Autodesk Inventor part; units mm, degrees
ref_plane "Work Plane1" through (-24.15, -24.15, 49.8) normal (0, 0, 1) x (1, 0, 0)
ref_plane "YZ Plane" through (0, 0, 0) normal (1, 0, 0) x (0, 1, 0)
ref_plane "XZ Plane" through (0, 0, 0) normal (0, 1, 0) x (-1, 0, 0)
sketch "Sketch1" plane through (0, 0, 0) normal (0, 0, 1) x (1, 0, 0)
  circle A0 centre (-21.9, -21.9) radius 1.875
  circle A1 centre (21.9, 21.9) radius 1.875
  circle A2 centre (21.9, -21.9) radius 1.875
  circle A3 centre (-21.9, 21.9) radius 1.875
  circle A4 centre (14.4, 20.8) radius 2.0675
  circle A5 centre (-14.4, -20.8) radius 2.0675
  circle A6 centre (14.4, -20.8) radius 2.0675
  circle A7 centre (20.8, -14.4) radius 2.0675
  line L0 (-17.05, 17.05) -> (-17.05, -17.05)
  line L1 (17.05, 17.05) -> (-17.05, 17.05)
  line L2 (17.05, -17.05) -> (17.05, 17.05)
  line L3 (-17.05, -17.05) -> (17.05, -17.05)
  circle A8 centre (20.8, 14.4) radius 2.0675
  circle A9 centre (-14.4, 20.8) radius 2.0675
  circle A10 centre (-20.8, -14.4) radius 2.0675
  circle A11 centre (-20.8, 14.4) radius 2.0675
  line L4 (-22.9, 24.15) -> (22.9, 24.15)
  arc A12 (-22.9, 24.15) -> (-24.15, 22.9) centre (-22.9, 22.9) ccw
  line L5 (-24.15, -22.9) -> (-24.15, 22.9)
  arc A13 (-24.15, -22.9) -> (-22.9, -24.15) centre (-22.9, -22.9) ccw
  line L6 (22.9, -24.15) -> (-22.9, -24.15)
  arc A14 (22.9, -24.15) -> (24.15, -22.9) centre (22.9, -22.9) ccw
  line L7 (24.15, 22.9) -> (24.15, -22.9)
  arc A15 (24.15, 22.9) -> (22.9, 24.15) centre (22.9, 22.9) ccw
  point P0 (0, 0)
ref_plane "Work Plane1" through (-24.15, -24.15, 49.8) normal (0, 0, 1) x (1, 0, 0)
extrude "Extrusion1" add sketch "Sketch1" along normal blind 1.5 from surface at 49.8 contours A0 | A1 | A2 | A3 | L1 L2 L3 L0 | L4 A15 L7 A14 L6 A13 L5 A12
sketch "Sketch2" plane through (-22.9, -24.15, 51.3) normal (0, 0, 1) x (1, 0, 0)
  arc A0 (-1.25, 1.25) -> (0, 0) centre (0, 1.25) ccw
  line L0 (45.8, 0) -> (0, 0)
  arc A1 (45.8, 0) -> (47.05, 1.25) centre (45.8, 1.25) ccw
  line L1 (47.05, 47.05) -> (47.05, 1.25)
  arc A2 (47.05, 47.05) -> (45.8, 48.3) centre (45.8, 47.05) ccw
  line L2 (0, 48.3) -> (45.8, 48.3)
  arc A3 (0, 48.3) -> (-1.25, 47.05) centre (0, 47.05) ccw
  line L3 (-1.25, 1.25) -> (-1.25, 47.05)
  circle A4 centre (2.1, 38.55) radius 2.0675
  circle A5 centre (2.1, 9.75) radius 2.0675
  circle A6 centre (8.5, 44.95) radius 2.0675
  circle A7 centre (43.7, 38.55) radius 2.0675
  circle A8 centre (43.7, 9.75) radius 2.0675
  circle A9 centre (37.3, 3.35) radius 2.0675
  circle A10 centre (8.5, 3.35) radius 2.0675
  circle A11 centre (37.3, 44.95) radius 2.0675
  arc A12 (47.9, 47.05) -> (45.8, 49.15) centre (45.8, 47.05) ccw
  line L4 (47.9, 47.05) -> (47.9, 1.25)
  arc A13 (45.8, -0.85) -> (47.9, 1.25) centre (45.8, 1.25) ccw
  line L5 (45.8, -0.85) -> (0, -0.85)
  arc A14 (-2.1, 1.25) -> (0, -0.85) centre (0, 1.25) ccw
  line L6 (-2.1, 1.25) -> (-2.1, 47.05)
  arc A15 (0, 49.15) -> (-2.1, 47.05) centre (0, 47.05) ccw
  line L7 (0, 49.15) -> (45.8, 49.15)
  line L8 (47.05, 1.25) -> (45.8, 1.25)
  line L9 (45.8, 1.25) -> (45.8, -0.85)
  line L10 (45.8, -0.85) -> (47.05, -0.85)
  line L11 (47.05, -0.85) -> (47.05, 1.25)
  line L12 (-1.25, 1.25) -> (0, 1.25)
  line L13 (0, 1.25) -> (0, -0.85)
  line L14 (0, -0.85) -> (-1.25, -0.85)
  line L15 (-1.25, -0.85) -> (-1.25, 1.25)
  line L16 (-1.25, 47.05) -> (0, 47.05)
  line L17 (0, 47.05) -> (0, 49.15)
  line L18 (0, 49.15) -> (-1.25, 49.15)
  line L19 (-1.25, 49.15) -> (-1.25, 47.05)
  line L20 (47.05, 47.05) -> (45.8, 47.05)
  line L21 (45.8, 47.05) -> (45.8, 49.15)
  line L22 (45.8, 49.15) -> (47.05, 49.15)
  line L23 (47.05, 49.15) -> (47.05, 47.05)
  point P0 (22.9, 24.15)
  dimension "d2" = 0.85
extrude "Extrusion2" add sketch "Sketch2" against normal blind 1.5 contours A0 L13 A14 L15 | L0 L9 L5 L13 | L19 A15 L17 A3 | A14 L14 L15 | A1 L11 A13 L9 | L17 L7 L21 L2 | L19 L18 A15 | A13 L11 L10 | L21 A12 L23 A2 | L22 L23 A12
pattern_linear "Rectangular Pattern1" count 2 spacing 50 along (0, 1, 0) of "Extrusion1", "Extrusion2"
chamfer "Chamfer1" distance 1.5 angle 45 2 edges at (0, -25, 51.3) (0, 75, 51.3)
properties part number "Panel Top 1x2"
Input: part model. Units: mm. Frame: model coordinates. Coordinates: 2 decimals unless noted, no trailing zeros. Order: outer loops, then holes, each group sorted by start corner. A loop starts at its lowest first (then second) coordinate and runs counter-clockwise, first axis right, second up. Notation, with made-up numbers: M -4.75,0.25 L 0.25,0.25 A16 ccw 0.25,24.25 Z; hole C -18.75,0 d4. An arc over 180 degrees is marked long. Write item = value, one per line. Start each with the question number.
(1) Section B-B on y = -20.8. Output: boundary loops of the cut face in (x, z), and give its area (3 significant figures).
(2) Pull-direction query (Y, two-part tool) for faces 1 (the flat face through (0, 26, 49.8)), 2 (the cylindrical face through (22.71, 15.19, 50.54)); classes: released by +Y, released by -Y, zero draft, split by the parting line, or undercut.
(3) Section A-A on x = -14.4. Give the number of separate pieces and of enclosed holes in the cut face, and give its area (3 significant figures).
(4) Line query: line 1 along X through (y, z) = (16, 50.05); line 2 along Y through (x, z) = (-14.4, 50.95); line 3 along Y through (x, z) = (-20.8, 50.95). Output: solid intervals per line, ascending. Write a range as [from, to].
(5) First-contact query: P1, Ø3.5, axis at x = 20.8, y = 14.4, coming from the -Z side; P2, Ø2, axis at x = 15.5, y = 30, coming from the +Z side. Flat tips, straight axial feed; report the tip coordinate or a pass-through.
Result set:
q1.outline = M -24.15,49.8 L -16.47,49.8 L -16.47,51.3 L -24.15,51.3 Z; M -12.33,49.8 L 12.33,49.8 L 12.33,51.3 L -12.33,51.3 Z; M 16.47,49.8 L 24.15,49.8 L 24.15,51.3 L 16.47,51.3 Z
q1.area = 60.0 mm²
q2.face_1 = zero draft
q2.face_2 = undercut
q3.separate_pieces = 5
q3.enclosed_holes = 0
q3.area = 123 mm²
q4.line_1 = [-24.15, -22.11], [-19.49, 19.49], [22.11, 24.15]
q4.line_2 = [-23.85, -22.87], [-18.73, 18.73], [22.87, 27.13], [31.27, 68.73], [72.87, 73.85]
q4.line_3 = [-23.85, -16.47], [-12.33, 12.33], [16.47, 33.53], [37.67, 62.33], [66.47, 73.85]
q5.P1 = through
q5.P2 = 51.3
